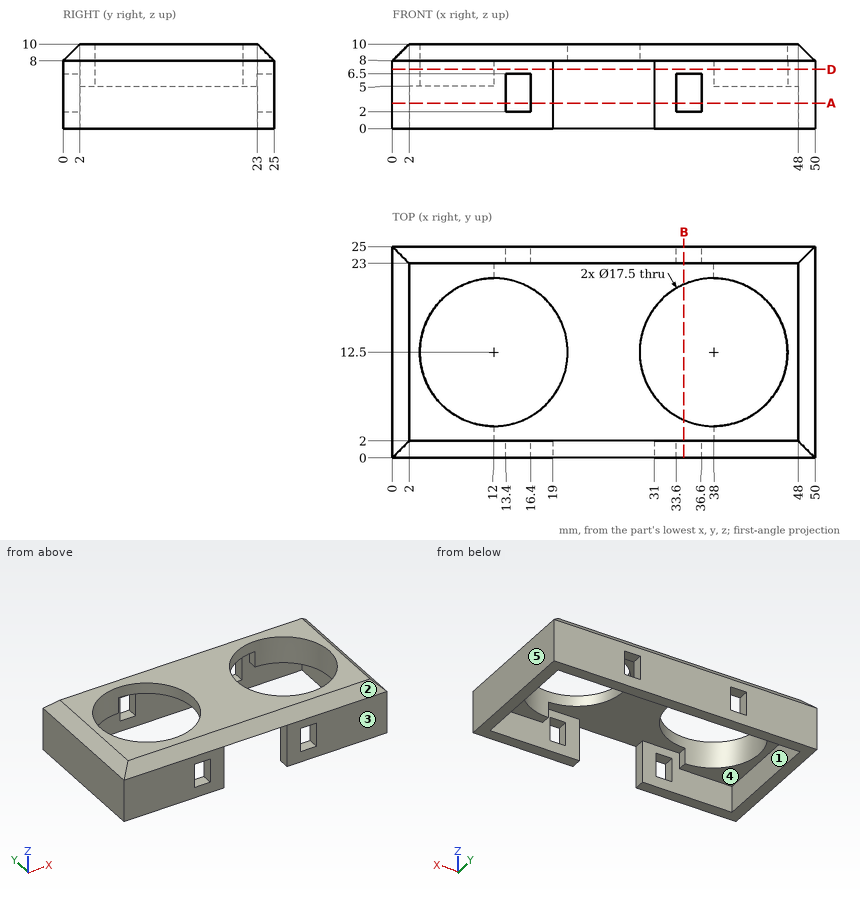
Geometry: see drawing. Coordinates: mm, zero at the bounding-box minimum. A direction names the side the tool comes from. Round coordinates to 2 decimals unless told otherwise and drop trailing zeros. Loops run counter-clockwise (first coordinate to the right, second up) from the corner with the lowest first, then second, coordinate; pieces in that order, holes last. Notation, with made-up numbers: M 37,10.25 L 42,10.25 A20 ccw 42,42.25 Z; hole C 75.25,0 d2. An arc over 180 degrees is marked long. Use a Markdown table: item, result. Add a question column.
1. Section query D-D on z = 7. Return the cut outline in (x, y).
2. Section query B-B on x = 34.5. Return the cut outline in (y, z), then the cut area to 3 significant figures.
3. Section query A-A on z = 3. Return the cut outline in (x, y), then the cut area to 3 significant figures.
4. Mould query, pull axis Y, two halves, no side actions, for the marked faces 3, 4 and 5. Classes: pulls with the +Y half, pulls with the -Y half, needs draft (parallel to the pull), parting line crosses it, or undercut.
5. Contact query for flat-ended pins moving along their axis: P1, Ø8, axis at x = 35, y = 11.5, coming from the -Z side; P2, Ø3, axis at x = 24.5, y = 8.5, coming from the -Z side. Output: stop coordinate, or through.
6. Line query: line 1 (Y direction, x = 3, z = 1.75); line 2 (X direction, y = 12.5, z = 7.2); line 3 (X direction, y = 5.25, z = 4.5). Output: solid intervals per line, ascending.
7. Reachability of the marked faces 1 and 2 from +Z, -Z, +X, -X, +Y, -Y: full face, straight path, thin tool, end or side. Return the list, or none.
Reported:
| question | item | result |
|---|---|---|
| 1 | outline | M 0,0 L 19,0 L 19,2 L 12,2 L 12,3.75 A8.75 cw 12,21.25 L 12,23 L 38,23 L 38,21.25 A8.75 cw 38,3.75 L 38,2 L 31,2 L 31,0 L 50,0 L 50,25 L 0,25 Z |
| 2 | outline | M 0,0 L 2,0 L 2,2 L 0,2 Z; M 0,6.5 L 2,6.5 L 2,8 L 4.48,8 L 4.48,10 L 2,10 L 0,8 Z; M 20.52,8 L 23,8 L 23,6.5 L 25,6.5 L 25,8 L 23,10 L 20.52,10 Z; M 23,0 L 25,0 L 25,2 L 23,2 Z |
| 2 | area | 27.9 mm² |
| 3 | outline | M 0,0 L 13.4,0 L 13.4,2 L 2,2 L 2,23 L 13.4,23 L 13.4,25 L 0,25 Z; M 16.4,0 L 19,0 L 19,2 L 16.4,2 Z; M 16.4,23 L 33.6,23 L 33.6,25 L 16.4,25 Z; M 31,0 L 33.6,0 L 33.6,2 L 31,2 Z; M 36.6,0 L 50,0 L 50,25 L 36.6,25 L 36.6,23 L 48,23 L 48,2 L 36.6,2 Z |
| 3 | area | 236 mm² |
| 4 | face 3 | pulls with the -Y half |
| 4 | face 4 | undercut |
| 4 | face 5 | needs draft |
| 5 | P1 | passes through |
| 5 | P2 | stops at z = 8 |
| 6 | line 1 | y = 0 to 2, 23 to 25 |
| 6 | line 2 | x = 0 to 3.25, 46.75 to 50 |
| 6 | line 3 | x = 0 to 2, 48 to 50 |
| 7 | face 1 | -Z |
| 7 | face 2 | +Z, +X, -X, -Y |
